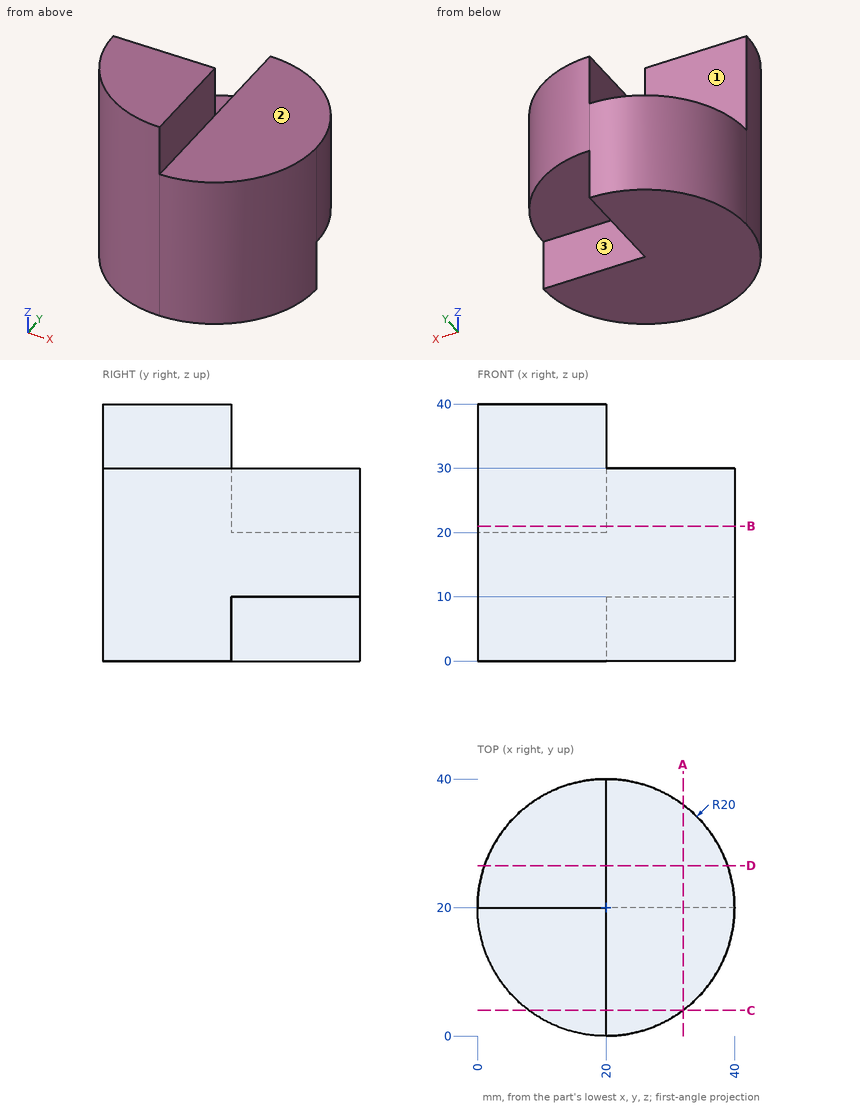
Drawing for the job (mm, zero at the part's lowest x, y, z). A direction names the side the tool comes from. Round coordinates to 2 decimals unless told otherwise and drop trailing zeros. Order: outer loops, then holes, each group sorted by start corner. A loop starts at its lowest first (then second) coordinate and runs counter-clockwise, first axis right, second up.
Item 1: Saw through at A-A on x = 32. Write the cut outline in (y, z).
Item 2: Saw through at D-D on y = 26.5. Write the cut outline in (x, z), then the cut area to 3 significant figures.
Item 3: Saw through at B-B on z = 21. Write the cut outline in (x, y).
Item 4: Pin check, flat tips, straight feed: pin 1 (8 mm diameter, centred on x = 7, z = 29.5, fed in from -Y); pin 2 (8 mm diameter, centred on x = 14.5, z = 24, fed in from -Y); pin 3 (1 mm diameter, centred on x = 12.5, z = 13, fed in from +Y) (3 decimals). Stop position of each tip, or through.
Item 5: Probe line 1 along Z through (x, y) = (8, 21.5); line 2 along Z through (x, y) = (21.5, 4); line 3 along Y through (x, z) = (38.5, 29). List the from-to ranges inside material, lowest first.
Item 6: Tool access for the marked faces 1, 2 and 3: list every direction of +Z, -Z, +X, -X, +Y, -Y with a clear straight run to the whole face (end or side of a thin tool).
Item 7: Saw through at C-C on y = 4. Write the cut outline in (x, z).
Reported:
1. outline: (4, 0) - (20, 0) - (20, 10) - (36, 10) - (36, 30) - (4, 30) - close
2. outline: (1.09, 0) - (20, 0) - (20, 10) - (38.91, 10) - (38.91, 30) - (20, 30) - (20, 20) - (1.09, 20) - close
2. area: 757 mm2
3. outline: (0, 20) arc R20 ccw (long way) to (20, 40) - (20, 20) - close
4. pin 1: stops at y = 2.14
4. pin 2: stops at y = 0.06
4. pin 3: stops at y = 38.735
5. line 1: z = 0 to 20
5. line 2: z = 0 to 30
5. line 3: y = 12.4 to 27.6
6. face 1: +Z, -X, +Y
6. face 2: +Z, +X, +Y, -Y
6. face 3: -Z, +X, +Y
7. outline: (8, 0) - (32, 0) - (32, 30) - (20, 30) - (20, 40) - (8, 40) - close
